Geometry check sheet. Reference: the model listing, model coordinates, mm. Give positions to 0.01 mm unless a question says otherwise; leave off trailing zeros. Order: outer loops, then holes, each group sorted by start corner. A loop starts at its lowest first (then second) coordinate and runs counter-clockwise, first axis right, second up.
from build123d import *

# Parameters (mm, degrees)
F0_W      = 2250
F0_H      = 250
F1_DEPTH  = 1.5
F3_D      = 11
F3_DEPTH  = 18
F3_TIP    = 3.3047334047
F5_DEPTH  = 3.001
F6_R      = 20
F7_DEPTH  = 3.001
F9_D      = 11
F9_DEPTH  = 18
F9_TIP    = 3.3047334047
F10_R     = 50
F11_W     = 200
F11_H     = 20
F12_DEPTH = 3.001


with BuildPart() as f1:
    # F0 (on Front) → F1 (new body, symmetric)
    with BuildSketch(Plane.XZ):
        Rectangle(F0_W, F0_H)
    extrude(amount=F1_DEPTH, both=True)

    # F3
    with Locations(Plane.XZ.offset(1.5)):
        with Locations((-1100, 56.2), (-1100, -100), (-925, -105.7), (-925, 45.1), (675, -28), (825, -28), (875, -105.7), (875, 45.1), (-475, 45.1), (-475, -105.7), (-25, -105.7), (-25, 45.1), (425, 45.1), (425, -105.7), (-825, -28), (-675, -28)):
            Hole(F3_D / 2, depth=F3_DEPTH)
            with Locations((0, 0, -(F3_DEPTH + F3_TIP / 2))):  # 118° drill point
                Cone(0, F3_D / 2, F3_TIP, mode=Mode.SUBTRACT)

    # F4 (on face) → F5 (cut, through all)
    with BuildSketch(Plane.XZ.offset(1.5)):
        with BuildLine():
            ThreePointArc((1110, 62), (1115.5, 67.5), (1110, 73))
            Line((1110, 73), (1090, 73))
            ThreePointArc((1090, 73), (1084.5, 67.5), (1090, 62))
            Line((1090, 62), (1110, 62))
        make_face()
        with BuildLine():
            ThreePointArc((1110, -38), (1115.5, -32.5), (1110, -27))
            Line((1110, -27), (1090, -27))
            ThreePointArc((1090, -27), (1084.5, -32.5), (1090, -38))
            Line((1090, -38), (1110, -38))
        make_face()
    extrude(amount=-F5_DEPTH, mode=Mode.SUBTRACT)

    # F6 (on face) → F7 (cut, through all)
    with BuildSketch(Plane.XZ.offset(1.5)):
        with Locations((1000, 17.5)):
            Circle(F6_R)
    extrude(amount=-F7_DEPTH, mode=Mode.SUBTRACT)

    # F9
    with Locations(Plane.XZ.offset(1.5)):
        with Locations((950.5, 17.5), (1049.5, 17.5)):
            Hole(F9_D / 2, depth=F9_DEPTH)
            with Locations((0, 0, -(F9_DEPTH + F9_TIP / 2))):  # 118° drill point
                Cone(0, F9_D / 2, F9_TIP, mode=Mode.SUBTRACT)

    # F10
    f10_edges = [f1.edges().sort_by_distance(p)[0] for p in [
        (1125, 0, 125),
        (1125, 0, -125),
    ]]
    fillet(f10_edges, radius=F10_R)

    # F11 (on face) → F12 (cut, through all)
    with BuildSketch(Plane.XZ.offset(1.5)):
        with Locations((-625, 115)):
            Rectangle(F11_W, F11_H)
    extrude(amount=-F12_DEPTH, mode=Mode.SUBTRACT)


solid = f1.part
Item 1: Scan lines: L1, parallel to Z at x = -27, y = 0.8; L2, parallel to Z at x = -475, y = -0.1; L3, parallel to Z at x = 1017.5, y = -0.6. Record each from-to range of solid material in increasing order.
Reported:
L1: z = -125 to -110.82, -100.58 to 39.98, 50.22 to 125
L2: z = -125 to -111.2, -100.2 to 39.6, 50.6 to 125
L3: z = -125 to 7.82, 27.18 to 125
Item 2: Sectioned sample at B-B (x = -638). Enter the section's corners in (y, z), and give its area (3 significant figures).
Reported:
outline: (-1.5, -125) - (1.5, -125) - (1.5, 105) - (-1.5, 105) - close
area: 690 mm2
Item 3: Draft check along X on faces 1 (the cylindrical face through (1109.964, 0.021, 110.742)), 2 (the cylindrical face through (1019.076, -0.021, 23.507)), 3 (the flat face through (-16, -1.5, 2)). Enter one of: released by +X, released by -X, zero draft, split by the parting line, or undercut.
Reported:
face 1: released by +X
face 2: undercut
face 3: zero draft
Item 4: Sectioned sample at A-A (y = 0.25). Give the number of separate pieces and of enclosed holes in the cut face, and give its area (3 significant figures).
Reported:
separate pieces: 1
enclosed holes: 21
area: 554,000 mm2
Item 5: Gauge pin test, flat ends, axial feed: pin 1 (1.5 mm diameter, centred on x = 1099.5, y = -0.5, fed in from -Z); pin 2 (1.5 mm diameter, centred on x = 1098, y = -0.5, fed in from +Z); pin 3 (1.5 mm diameter, centred on y = -0.5, z = 111.5, fed in from +X). Record the tip position at first contact, or that the pin passes through.
Reported:
pin 1: stops at z = -119
pin 2: stops at z = 119.78
pin 3: stops at x = 1109.96
